Verification items for the finished model (mm, model axes). A direction names the side the tool comes from. Round coordinates to 2 decimals unless told otherwise and drop trailing zeros. Write each loop counter-clockwise with the first axis right and the second up, starting at its lowest first coordinate (ties: lowest second). Pieces come first, ordered by that corner, then holes. Notation, with made-up numbers: (15, 5) - (43, 5) arc R23 ccw to (43, 40) - close; hole circle Ø4 at (65.25, 14.25). An arc over 180 degrees is marked (long way). Answer as a JSON object with one key per item and string values.
```python
from build123d import *

# Parameters (mm, degrees)
SKETCH1_W           = 100
SKETCH1_H           = 24
SKETCH1_R           = 3.5
BOSS_EXTRUDE1_DEPTH = 5
BOSS_EXTRUDE2_DEPTH = 9
SKETCH3_R           = 8
CUT_EXTRUDE1_DEPTH  = 10


with BuildPart() as part:
    # Sketch1 → Boss-Extrude1 (new body)
    with BuildSketch(Plane(origin=(0, 0, 0), x_dir=(1, 0, 0), z_dir=(0, 1, 0))):
        Rectangle(SKETCH1_W, SKETCH1_H)
        with Locations((-45, 7)):
            Circle(SKETCH1_R, mode=Mode.SUBTRACT)
        with Locations((-45, -7)):
            Circle(SKETCH1_R, mode=Mode.SUBTRACT)
        with Locations((45, 7)):
            Circle(SKETCH1_R, mode=Mode.SUBTRACT)
        with Locations((45, -7)):
            Circle(SKETCH1_R, mode=Mode.SUBTRACT)
    extrude(amount=BOSS_EXTRUDE1_DEPTH)

    # Sketch2 → Boss-Extrude2 (add)
    with BuildSketch(Plane.XY.offset(3)):
        with BuildLine():
            Line((-29.978021695, 5), (29.763516014, 5))
            Line((29.763516014, 5), (11.035619534, 51.854874594))
            ThreePointArc((11.035619534, 51.854874594), (-0.107252841, 59.401067767), (-11.250125215, 51.854874594))
            Line((-11.250125215, 51.854874594), (-29.978021695, 5))
        make_face()
    extrude(amount=BOSS_EXTRUDE2_DEPTH)

    # Sketch3 → Cut-Extrude1 (cut, through all)
    with BuildSketch(Plane(origin=(0, 0, 3), x_dir=(-1, 0, 0), z_dir=(0, 0, -1))):
        with Locations((0, 49.578279074)):
            Circle(SKETCH3_R)
    extrude(amount=-CUT_EXTRUDE1_DEPTH, mode=Mode.SUBTRACT)


solid = part.part
```
Q1. Release check for a two-part mould opening along Z. For faces 3 (the cylindrical face through (41.503, 2.465, -7.154)), 4 (the cylindrical face through (0.1, 59.4, 7.4)), 5 (the flat face through (-1, 2, -12)), 6 (the flat face through (-1, 16, 12)) record: released by +Z, released by -Z, zero draft, split by the parting line, or undercut.
Geometry check:
{"face 3": "undercut", "face 4": "zero draft", "face 5": "released by -Z", "face 6": "released by +Z"}
Q2. Section check C-C, the plane z = -7. Record the cut outline in (x, y), then the cut area to 3 significant figures.
Geometry check:
{"outline": "(-50, 0) - (-48.5, 0) - (-48.5, 5) - (-50, 5) - close; (-41.5, 0) - (41.5, 0) - (41.5, 5) - (-41.5, 5) - close; (48.5, 0) - (50, 0) - (50, 5) - (48.5, 5) - close", "area": "430 mm2"}
Q3. Set-up check for faces 1 (the flat face through (-1, 27, 3)), 2 (the cylindrical face through (41.503, 2.465, 6.846)): record each of +Z, -Z, +X, -X, +Y, -Y from which the full face is reachable in a straight line by a thin tool's end or side.
Geometry check:
{"face 1": "-Z, +X, -X, +Y", "face 2": "+Y, -Y"}
Q4. Section check B-B, the plane z = 6. Record the cut outline in (x, y).
Geometry check:
{"outline": "(-50, 0) - (-48.35, 0) - (-48.35, 5) - (-50, 5) - close; (-41.65, 0) - (41.65, 0) - (41.65, 5) - (29.76, 5) - (11.04, 51.85) arc R12 ccw to (-11.25, 51.85) - (-29.98, 5) - (-41.65, 5) - close; (48.35, 0) - (50, 0) - (50, 5) - (48.35, 5) - close; hole circle Ø16 at (0, 49.58)"}
Q5. Section check D-D, the plane x = 0. Record the cut outline in (y, z).
Geometry check:
{"outline": "(0, -12) - (5, -12) - (5, 3) - (41.58, 3) - (41.58, 12) - (0, 12) - close; (57.58, 3) - (59.4, 3) - (59.4, 12) - (57.58, 12) - close"}
Q6. Section check A-A, the plane x = -45. Record the cut outline in (y, z).
Geometry check:
{"outline": "(0, -12) - (5, -12) - (5, -10.5) - (0, -10.5) - close; (0, -3.5) - (5, -3.5) - (5, 3.5) - (0, 3.5) - close; (0, 10.5) - (5, 10.5) - (5, 12) - (0, 12) - close"}
Q7. Gauge pin test, flat ends, axial feed: P1, Ø12, axis at x = -1.5, z = -1.5, coming from the +Y side; P2, Ø6, axis at x = -17.5, y = 14, coming from the -Z side; P3, Ø9, axis at x = 45, z = 7, coming from the +Y side; P4, Ø6, axis at y = 37, z = -1.5, coming from the -X side. Record the tip position at first contact, or that the pin passes through.
Geometry check:
{"P1": "stops at y = 59.4", "P2": "stops at z = 3", "P3": "stops at y = 5", "P4": "passes through"}
Q8. Material ranges on line 1 along Z through (x, y) = (-45, 2.7); line 2 along X through (y, z) = (3.25, 7); line 3 along Y through (x, z) = (0, 5.75), recorded low to high. Write a range as [from, to].
Geometry check:
{"line 1": "z = [-12, -10.5], [-3.5, 3.5], [10.5, 12]", "line 2": "x = [-50, -48.5], [-41.5, 41.5], [48.5, 50]", "line 3": "y = [0, 41.58], [57.58, 59.4]"}
